from build123d import *

# Parameters (mm, degrees)
F0_R     = 40
F0_R_2   = 39
F1_DEPTH = 200


# Not quite as in the source:
# - a fillet or chamfer that OpenCascade refuses, or shapes differently, is made with other operations: its cross-section is extruded or revolved along the edge and cut away or added


with BuildPart() as f1:
    # F0 (on Front) → F1 (new body)
    with BuildSketch(Plane.XZ):
        Circle(F0_R)
        Circle(F0_R_2, mode=Mode.SUBTRACT)
    extrude(amount=F1_DEPTH)

    # F2 (on Right) → F3 (revolve)
    with BuildSketch(Plane.YZ):
        Polygon((0, 0), (0, -39.8333705962), (3, -39.8333705962), (6, 0), align=None)
    revolve(axis=Axis((0, 3, 0), (0, -1, 0)))

    # F4: fillet of radius 5 on 1 edges, made by hand

    # F4_s1 → F4_t2 (revolve, cut)
    with BuildSketch(Plane.YZ):
        with BuildLine():
            ThreePointArc((0.000132768, -39.8337479192), (2.3100716804, -38.1578030018), (3.3274101289, -35.4914137529))
            Line((3.3274101289, -35.4914137529), (3.8261475828, -35.5289755344))
            ThreePointArc((3.8261475828, -35.5289755344), (3.6622430832, -37.6999389358), (3.4987374539, -39.8709323776))
            Line((3.4987374539, -39.8709323776), (3, -40.3335205091))
            ThreePointArc((3, -40.3335205091), (1.500066384, -40.3335205091), (0.1661424858, -40.3055431173))
            Line((0.1661424858, -40.3055431173), (0.000132768, -39.8337479192))
        make_face()
    revolve(axis=Axis((0, 3, 0), (0, -1, 0)), mode=Mode.SUBTRACT)


solid = f1.part
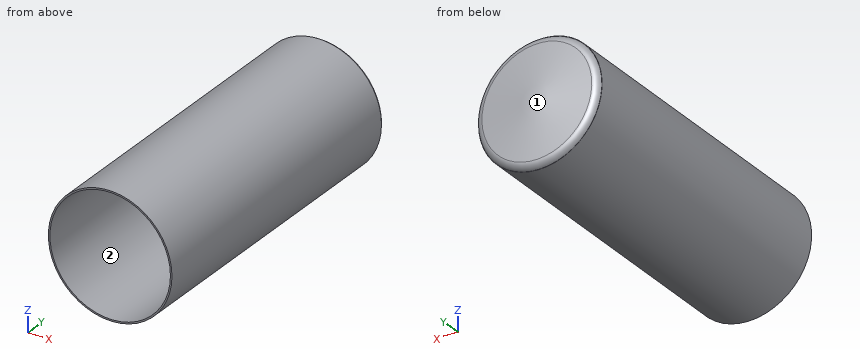
Check sheet for the modelled part. Datum: model origin and axes. Units: mm. Face numbers are marked on the shaded views. Round coordinates to 2 decimals unless told otherwise and drop trailing zeros. Loops run counter-clockwise (first coordinate to the right, second up) from the corner with the lowest first, then second, coordinate; pieces in that order, holes last.
1. Mould release check, pull along Z, two halves, no side actions. Record for the marked faces 1 and 2: released by +Z, released by -Z, zero draft, split by the parting line, or undercut.
2. Scan lines: probe 1 along Z at (x, y) = (0, -107); probe 2 along X at (y, z) = (-65, -35.5); probe 3 along X at (y, z) = (-103, -19). Record each from-to range of solid material in increasing order.
3. Sectioned sample at A-A on y = -37. Record the boundary of the cut face in (x, z).
4. Gauge pin test, flat ends, axial feed: pin 1 Ø3 at (x, y) = (-1, -132) entering from -Z; pin 2 Ø1.5 at (y, z) = (-146, 4.5) entering from +X; pin 3 Ø10 at (y, z) = (-122, -10.5) entering from -X. Record the tip position at first contact, or that the pin passes through.
Recorded:
1. face 1: split by the parting line
1. face 2: undercut
2. probe 1: z = -40 to -39, 39 to 40
2. probe 2: x = -18.43 to -16.15, 16.15 to 18.43
2. probe 3: x = -35.2 to -34.06, 34.06 to 35.2
3. outline: circle Ø80 at (0, 0); hole circle Ø78 at (0, 0)
4. pin 1: stops at z = -40
4. pin 2: stops at x = 39.82
4. pin 3: stops at x = -39.62
